from build123d import *

# Parameters (mm, degrees)
F0_W          = 120
F0_H          = 80
F1_DEPTH      = 25.4
F1_DEPTH_BACK = 25.4
F3_D          = 50.8
F5_D          = 25.4
F7_D          = 25.4


with BuildPart() as f1:
    # F0 (on Top) → F1 (new body, two sides)
    with BuildSketch(Plane.XY) as f1_sk:
        Rectangle(F0_W, F0_H)
    extrude(amount=F1_DEPTH)
    extrude(f1_sk.sketch, amount=-F1_DEPTH_BACK)

    # F3 (through all)
    with Locations(Plane.XY.offset(25.4)):
        with Locations((0, 0)):
            Hole(F3_D / 2)

    # F5 (through all)
    with Locations(Plane.XZ.offset(40)):
        with Locations((0, 0)):
            Hole(F5_D / 2)

    # F7 (through all)
    with Locations(Plane(origin=(-60, 0, 0), x_dir=(0, -1, 0), z_dir=(-1, 0, 0))):
        with Locations((0, 0)):
            Hole(F7_D / 2)


solid = f1.part
Geometry: final body of the model. Coordinates: model frame, mm. Coordinates: 2 decimals unless noted, no trailing zeros. Loops run counter-clockwise (first coordinate to the right, second up) from the corner with the lowest first, then second, coordinate; pieces in that order, holes last. Notation, with made-up numbers: (76, -22.5) - (135, -22.5) arc R30 ccw to (135, 6.5) - close; hole circle Ø10 at (-32, 72.5). An arc over 180 degrees is marked (long way). One line per question, with ' | ' between items. Start each with the question number.
(1) Cut plane D-D on y = 20. Output: boundary loops of the cut face in (x, z), and give its area (3 significant figures).
(2) First-contact query: pin 1 (20.5 mm diameter, centred on y = 0, z = 0, fed in from -X). Flat tip, straight axial feed; report the tip coordinate or a pass-through.
(3) Cut plane A-A on z = 0. Output: boundary loops of the cut face in (x, y), and give its area (3 significant figures).
(4) Cut plane C-C on x = 0. Output: boundary loops of the cut face in (y, z).
(5) Ray query, L1, parallel to X at y = -34.75, z = 0; L2, parallel to Z at x = 0, y = 28.5; L3, parallel to Z at x = 2, y = -34.5. Return the intervals inside material, ascending. Write a range as from..to.
(6) Cut plane B-B on y = 0. Output: boundary loops of the cut face in (x, z).
(7) Draft query along Y for faces 1 (the flat face through (-14, -40, 0)), 2 (the cylindrical face through (41.265, -12.688, 0.558)), 3 (the flat face through (-28, 1, -25.4)). Return one class per face: +Y half, -Y half, draft (parallel to the pull), parting line (faces both ways), or undercut.
Here are the results:
1) outline: (-60, -25.4) - (-15.66, -25.4) - (-15.66, 25.4) - (-60, 25.4) - close; (15.66, -25.4) - (60, -25.4) - (60, 25.4) - (15.66, 25.4) - close | area: 4,510 mm²
2) pin 1: through
3) outline: (-60, -40) - (-12.7, -40) - (-12.7, -22) arc R25.4 cw to (-22, -12.7) - (-60, -12.7) - close; (-60, 12.7) - (-22, 12.7) arc R25.4 cw to (-12.7, 22) - (-12.7, 40) - (-60, 40) - close; (12.7, -40) - (60, -40) - (60, -12.7) - (22, -12.7) arc R25.4 cw to (12.7, -22) - close; (12.7, 22) arc R25.4 cw to (22, 12.7) - (60, 12.7) - (60, 40) - (12.7, 40) - close | area: 4,960 mm²
4) outline: (-40, -25.4) - (-25.4, -25.4) - (-25.4, -12.7) - (-40, -12.7) - close; (-40, 12.7) - (-25.4, 12.7) - (-25.4, 25.4) - (-40, 25.4) - close; (25.4, -25.4) - (40, -25.4) - (40, -12.7) - (25.4, -12.7) - close; (25.4, 12.7) - (40, 12.7) - (40, 25.4) - (25.4, 25.4) - close
5) L1: -60..-12.7, 12.7..60 | L2: -25.4..-12.7, 12.7..25.4 | L3: -25.4..-12.54, 12.54..25.4
6) outline: (-60, -25.4) - (-25.4, -25.4) - (-25.4, -12.7) - (-60, -12.7) - close; (-60, 12.7) - (-25.4, 12.7) - (-25.4, 25.4) - (-60, 25.4) - close; (25.4, -25.4) - (60, -25.4) - (60, -12.7) - (25.4, -12.7) - close; (25.4, 12.7) - (60, 12.7) - (60, 25.4) - (25.4, 25.4) - close
7) face 1: -Y half | face 2: undercut | face 3: draft
